from build123d import *

# Parameters (mm, degrees)
SKETCH1_R           = 9
BOSS_EXTRUDE1_DEPTH = 8.8
SKETCH2_W           = 4.5
SKETCH2_H           = 4.4
CUT_EXTRUDE1_DEPTH  = 10


with BuildPart() as part:
    # Sketch1 → Boss-Extrude1 (new body)
    with BuildSketch(Plane(origin=(0, 0, 0), x_dir=(1, 0, 0), z_dir=(0, 1, 0))):
        Circle(SKETCH1_R)
        with BuildLine():
            ThreePointArc((5.95, 0), (-3.317755265, -4.939129478), (-2.25, 5.508175742))
            Line((-2.25, 5.508175742), (-2.25, 7.508175742))
            Line((-2.25, 7.508175742), (2.25, 7.508175742))
            Line((2.25, 7.508175742), (2.25, 5.508175742))
            ThreePointArc((2.25, 5.508175742), (4.939129478, 3.317755265), (5.95, 0))
        make_face(mode=Mode.SUBTRACT)
    extrude(amount=BOSS_EXTRUDE1_DEPTH)

    # Sketch2 → Cut-Extrude1 (cut, through all)
    with BuildSketch(Plane.XY):
        with Locations((0, 6.6)):
            Rectangle(SKETCH2_W, SKETCH2_H)
    extrude(amount=-CUT_EXTRUDE1_DEPTH, mode=Mode.SUBTRACT)


solid = part.part
Source: CAD feature listing. Evaluate the final solid. Frame: model axes, mm. A direction names the side the tool comes from. Round coordinates to 2 decimals unless told otherwise and drop trailing zeros. Write each loop counter-clockwise with the first axis right and the second up, starting at its lowest first coordinate (ties: lowest second). Pieces come first, ordered by that corner, then holes. Notation, with made-up numbers: M 15.5,23 L 48.5,23 A24 ccw 48.5,34 Z; hole C 47,46 d7. An arc over 180 degrees is marked long. One line per item, written item: value. Start each with the question number.
Item 1: Section query A-A (x = 0). Return the cut outline in (y, z).
Item 2: Mould query, pull axis Z, two halves, no side actions, for faces 1 (the flat face through (2, 8.8, 6)), 2 (the cylindrical face through (-1.951, 4.338, 8.786)), 3 (the flat face through (2.25, 4, -7)). Classes: pulls with the +Z half, pulls with the -Z half, needs draft (parallel to the pull), parting line crosses it, or undercut.
Item 3: Section query D-D (y = 5). Return the cut outline in (x, z), plus the area to 3 significant figures.
Item 4: Section query B-B (y = 3). Return the cut outline in (x, z), plus the area to 3 significant figures.
Item 5: Section query C-C (z = 4). Return the cut outline in (x, y).
Item 6: Pin query (flat end, axial travel): pin 1 (2 mm diameter, centred on x = -7, z = -6.5, fed in from -Y); pin 2 (1 mm diameter, centred on y = 4, z = -7.5, fed in from -X); pin 3 (1.6 mm diameter, centred on x = 0.5, z = -8.5, fed in from +Y); pin 4 (4 mm diameter, centred on x = 2.5, y = 5.5, fed in from +Z). Return the tip coordinate at first contact, or that it passes through.
Item 7: Ray query, L1, parallel to X at y = 5.75, z = 0; L2, parallel to Z at x = 0.25, y = 3.25; L3, parallel to Z at x = 0, y = 5.75. Return the intervals inside material, ascending. Write a range as from..to.
Item 8: Set-up query: faces 4 (the flat face through (0, 2, -7.508)), 5 (the flat face through (2, 0, 6)), 6 (the flat face through (0, 4.4, -8)), 7 (the flat face through (-2.25, 4, -7)). Return all of +Z, -Z, +X, -X, +Y, -Y with unobstructed straight access to the full face (end or side cutting, diameter ignored); none if empty.
Result set:
1. outline: M 0,-9 L 4.4,-9 L 4.4,-7.51 L 0,-7.51 Z; M 0,5.95 L 8.8,5.95 L 8.8,9 L 0,9 Z
2. face 1: needs draft
2. face 2: parting line crosses it
2. face 3: undercut
3. outline: M -2.25,-8.71 L -2.25,-5.51 A5.95 cw long 2.25,-5.51 L 2.25,-8.71 A9 ccw long Z
3. area: 129 mm²
4. outline: C 0,0 d18; hole M -2.25,-7.51 L 2.25,-7.51 L 2.25,-5.51 A5.95 ccw long -2.25,-5.51 Z
4. area: 136 mm²
5. outline: M -8.06,0 L -4.4,0 L -4.4,8.8 L -8.06,8.8 Z; M 4.4,0 L 8.06,0 L 8.06,8.8 L 4.4,8.8 Z
6. pin 1: stops at y = 0
6. pin 2: stops at x = -5.66
6. pin 3: stops at y = 4.4
6. pin 4: stops at z = 8.99
7. L1: x = -9..-5.95, 5.95..9
7. L2: z = -9..-7.51, 5.94..9
7. L3: z = 5.95..9
8. face 4: +Y, -Y
8. face 5: +Z, -Z, +X, -X, -Y
8. face 6: -Z, +Y
8. face 7: +Y
